Can you work these out from the model? Positions are in its coordinate system, mm. A direction names the side the tool comes from. Coordinates: 2 decimals unless noted, no trailing zeros. Order: outer loops, then holes, each group sorted by start corner. A loop starts at its lowest first (then second) coordinate and runs counter-clockwise, first axis right, second up. Notation, with made-up numbers: (12.25, 71.5) -> (62.25, 71.5) arc R23 ccw to (62.25, 99.5) -> close; hole circle Ø1 at (-40, 2.5). An arc over 180 degrees is marked (long way). Answer in a Markdown table with one row per item.
Autodesk Inventor part; units mm, degrees
ref_plane "Work Plane1" through (26.995, -107.2374, 17.5) normal (0, 0, -1) x (0.0784, 0.9969, 0)
ref_plane "YZ Plane" through (0, 0, 0) normal (1, 0, 0) x (0, 1, 0)
ref_plane "XZ Plane" through (0, 0, 0) normal (0, 1, 0) x (-1, 0, 0)
sketch "Sketch1" plane through (0, 0, 0) normal (0, 0, 1) x (1, 0, 0)
  line L0 (9.525, -19.05) -> (-9.525, -19.05)
  line L1 (-9.525, -19.05) -> (-9.525, 19.05)
  line L2 (-9.525, 19.05) -> (9.525, 19.05)
  line L3 (9.525, 19.05) -> (9.525, -19.05)
  line L4 (9.525, -19.05) -> (-9.525, 19.05) construction
  line L5 (-9.525, -19.05) -> (9.525, 19.05) construction
  line L6 (19.525, -29.05) -> (-19.525, -29.05)
  line L7 (-19.525, -29.05) -> (-19.525, 29.05)
  line L8 (-19.525, 29.05) -> (19.525, 29.05)
  line L9 (19.525, 29.05) -> (19.525, -29.05)
  line L10 (19.525, -29.05) -> (-19.525, 29.05) construction
  line L11 (-19.525, -29.05) -> (19.525, 29.05) construction
  line L12 (-19.525, 0) -> (-59.525, 0) construction
  circle A0 centre (-59.525, 0) radius 4
  line L13 (-59.525, 0) -> (-19.525, 0) construction
  line L14 (-59.525, -10) -> (-19.525, -10)
  line L15 (-19.525, 10) -> (-59.525, 10)
  arc A1 (-59.525, 10) -> (-59.525, -10) centre (-59.525, 0) ccw
  arc A2 (-19.525, -10) -> (-19.525, 10) centre (-19.525, 0) ccw construction
  line L16 (-19.525, 10) -> (-19.525, -10)
  point P0 (0, 0)
  point P1 (-39.525, 0)
  dimension "d0" = 38.1
  dimension "d1" = 19.05
  dimension "d2" = 10
  dimension "d3" = 10
  dimension "d4" = 8
  dimension "d5" = 10
  dimension "d6" = 40
extrude "Extrusion1" add sketch "Sketch1" along normal blind 15
sketch "Sketch2" plane through (0, 0, 15) normal (0, 0, 1) x (1, 0, 0)
  line L0 (-9.525, -19.05) -> (-9.525, 19.05)
  line L1 (-9.525, 19.05) -> (9.525, 19.05)
  line L2 (9.525, 19.05) -> (9.525, -19.05)
  line L3 (9.525, -19.05) -> (-9.525, -19.05)
  circle A0 centre (-59.525, 0) radius 4
  line L4 (-59.525, -10) -> (-19.525, -10)
  line L5 (-19.525, -10) -> (-19.525, -29.05)
  line L6 (-19.525, -29.05) -> (19.525, -29.05)
  line L7 (19.525, -29.05) -> (19.525, 29.05)
  line L8 (19.525, 29.05) -> (-19.525, 29.05)
  line L9 (-19.525, 29.05) -> (-19.525, 10)
  line L10 (-19.525, 10) -> (-59.525, 10)
  arc A1 (-59.525, 10) -> (-59.525, -10) centre (-59.525, 0) ccw
  point P0 (0, 0)
extrude "Extrusion2" add sketch "Sketch2" along normal blind 5 contours L0 L1 L2 L3 | A1 L10 L9 L8 L7 L6 L5 L4
sketch "Sketch3" plane through (0, 0, 15) normal (0, 0, -1) x (-1, 0, 0)
  circle A0 centre (0, 0) radius 2.5
  dimension "d11" = 5
extrude "Extrusion3" cut sketch "Sketch3" against normal through all
sketch "Sketch4" plane through (0, 0, 20) normal (0, 0, 1) x (1, 0, 0)
  line L0 (0, 0) -> (45, 0) construction
  line L1 (45, 0) -> (45, -80) construction
  line L2 (45, -80) -> (0, -80) construction
  line L3 (0, -80) -> (0, 0) construction
  circle A0 centre (45, -80) radius 4.25
  line L4 (19.525, -29.05) -> (-19.525, -29.05) construction
  line L5 (19.525, -29.05) -> (9.525, -29.05) construction
  line L6 (9.525, -29.05) -> (9.525, -19.05) construction
  line L7 (9.525, -19.05) -> (19.525, -19.05) construction
  line L8 (19.525, -19.05) -> (19.525, -29.05) construction
  line L9 (9.525, -19.05) -> (45, -80) construction
  line L10 (1.5305, -23.7031) -> (37.0055, -84.6531)
  line L11 (52.9945, -75.3469) -> (17.5195, -14.3969)
  arc A1 (17.5195, -14.3969) -> (1.5305, -23.7031) centre (9.525, -19.05) ccw
  arc A2 (37.0055, -84.6531) -> (52.9945, -75.3469) centre (45, -80) ccw
  point P0 (27.2625, -49.525)
  dimension "d14" = 80
  dimension "d15" = 45
  dimension "d16" = 8.5
  dimension "d17" = 10
  dimension "d18" = 10
  dimension "d19" = 5
ref_plane "Work Plane1" through (26.995, -107.2374, 17.5) normal (0, 0, -1) x (0.0784, 0.9969, 0)
extrude "Extrusion4" add sketch "Sketch4" along normal up to surface (17.5 mm away) from surface at -20
sketch "Sketch5" plane through (0, 0, 0) normal (0, 0, -1) x (-1, 0, 0)
  circle A0 centre (-45, -80) radius 4.25
  line L0 (-9.525, -9.8) -> (-9.525, 19.05)
  line L1 (-9.525, 19.05) -> (9.525, 19.05)
  line L2 (9.525, 19.05) -> (9.525, -19.05)
  line L3 (9.525, -19.05) -> (-0.275, -19.05)
  arc A1 (-0.275, -19.05) -> (-9.525, -9.8) centre (-9.525, -19.05) ccw
  line L4 (-19.525, -17.8427) -> (-52.9945, -75.3469)
  arc A2 (-52.9945, -75.3469) -> (-37.0055, -84.6531) centre (-45, -80) ccw
  line L5 (-37.0055, -84.6531) -> (-4.6426, -29.05)
  line L6 (-4.6426, -29.05) -> (19.525, -29.05)
  line L7 (19.525, -29.05) -> (19.525, -10)
  line L8 (59.525, -10) -> (19.525, -10)
  arc A3 (59.525, -10) -> (59.525, 10) centre (59.525, 0) ccw
  line L9 (19.525, 10) -> (59.525, 10)
  line L10 (19.525, 10) -> (19.525, 29.05)
  line L11 (19.525, 29.05) -> (-19.525, 29.05)
  line L12 (-19.525, 29.05) -> (-19.525, -17.8427)
  circle A4 centre (59.525, 0) radius 4
  arc A5 (-0.275, -19.05) -> (-9.525, -9.8) centre (-9.525, -19.05) ccw
  line L13 (-0.275, -19.05) -> (-9.525, -19.05)
  line L14 (-9.525, -19.05) -> (-9.525, -9.8)
  line L15 (-9.525, -9.8) -> (-0.275, -9.8)
  line L16 (-0.275, -9.8) -> (-0.275, -19.05)
  point P0 (0, 0)
extrude "Extrusion5" cut sketch "Sketch5" against normal up to surface (15 mm away) contours L15 L16 A1 | A1 L13 L14
properties part number "tiller frame bracket"
(1) Suppose I cut it at C-C (x = 45). Please give me the cut outline in (y, z), and give its area (3 significant figures).
Response values:
| item | result |
|---|---|
| outline | (-89.25, 0) -> (-84.25, 0) -> (-84.25, 17.5) -> (-89.25, 17.5) -> close; (-75.75, 0) -> (-61.61, 0) -> (-61.61, 17.5) -> (-75.75, 17.5) -> close |
| area | 335 mm2 |
(2) Suppose I cut it at B-B (z = 9.25). Count the separate pieces of the cut face and the enclosed holes in it, and give its area (3 significant figures).
Response values:
| item | result |
|---|---|
| separate pieces | 1 |
| enclosed holes | 3 |
| area | 3,650 mm2 |
(3) Suppose I cut it at D-D (y = -80). Please give me the cut outline in (x, z), and give its area (3 significant figures).
Response values:
| item | result |
|---|---|
| outline | (34.3, 0) -> (40.75, 0) -> (40.75, 17.5) -> (34.3, 17.5) -> close; (49.25, 0) -> (54.25, 0) -> (54.25, 17.5) -> (49.25, 17.5) -> close |
| area | 200 mm2 |
(4) I need wall thicknesses on line 1 (Y direction, x = 0, z = 16.5); line 2 (Y direction, x = 0.5, z = 5.25); line 3 (X direction, y = 3, z = 11) (3 decimals). Which ranges of each line are inside material? Lowest first, please. Write a range as [from, to].
Response values:
| item | result |
|---|---|
| line 1 | [-29.05, -2.5], [2.5, 29.05] |
| line 2 | [-29.05, -19.05], [19.05, 29.05] |
| line 3 | [-69.064, -62.171], [-56.879, -9.525], [9.525, 19.525] |
(5) Will these pins go through, and if not, where does the flat tip stop? pin 1 Ø7.5 at (y, z) = (-14.5, 7.5) entering from -X (3 decimals); pin 2 Ø12 at (x, z) = (-3, 8) entering from -Y; pin 3 Ø25 at (x, y) = (36.5, -36.5) entering from +Z; pin 4 Ø3 at (x, y) = (0, 0) entering from +Z.
Response values:
| item | result |
|---|---|
| pin 1 | x = -19.525 |
| pin 2 | y = -29.05 |
| pin 3 | z = 17.5 |
| pin 4 | through |
(6) Suppose I cut it at A-A (y = 0). Please give me the cut outline in (x, z) (3 decimals), and give its area (3 significant figures).
Response values:
| item | result |
|---|---|
| outline | (-69.525, 0) -> (-63.525, 0) -> (-63.525, 20) -> (-69.525, 20) -> close; (-55.525, 0) -> (-9.525, 0) -> (-9.525, 15) -> (-2.5, 15) -> (-2.5, 20) -> (-55.525, 20) -> close; (2.5, 15) -> (9.525, 15) -> (9.525, 0) -> (19.525, 0) -> (19.525, 20) -> (2.5, 20) -> close |
| area | 1,310 mm2 |
(7) On a 3-axis mill with a long thin cutter (end or side, diameter ignored), from which of +Z, -Z, +X, -X, +Y, -Y can I reach the whole of each face in a straight line? I mean faces 1 (the cylindrical face through (-69.523, -0.22, 9.86)), 2 (the flat face through (-19.525, -20, 10)), 3 (the flat face through (-39, 10, 10)), 4 (the flat face through (4, 0, 15)), 5 (the cylindrical face through (-63.52, -0.18, 9.86)). Say none if no direction works.
Response values:
| item | result |
|---|---|
| face 1 | +Z, -Z, -X |
| face 2 | +Z, -Z, -X, -Y |
| face 3 | +Z, -Z, -X, +Y |
| face 4 | -Z |
| face 5 | +Z, -Z |
